Can you work these out from the model? Positions are in its coordinate system, mm. A direction names the side the tool comes from. Coordinates: 2 decimals unless noted, no trailing zeros. Order: outer loops, then holes, each group sorted by start corner. A loop starts at its lowest first (then second) coordinate and runs counter-clockwise, first axis right, second up. Notation, with made-up numbers: M -34,56.5 L 25,56.5 A33 ccw 25,92.5 Z; hole C 52,67 d3. An arc over 180 degrees is marked long. Answer as CSV lines item,"result". Start each with the question number.
1. If we mould it in two halves opening along Z, with no side actions, what happens to faces 1 (the face through (9.05, 16.44, -9.07)), 2 (the face through (0, 31, 0.794)), 3 (the face through (9.07, 16.44, 9.05)), 4 (the face through (2, 0, 0))? For each: released by +Z, released by -Z, zero draft, split by the parting line, or undercut.
2. On a 3-axis mill with a long thin cutter (end or side, diameter ignored), from which of +Z, -Z, +X, -X, +Y, -Y can I reach the whole of each face in a straight line? I mean faces 5 (the face through (2, 27, 4.762)), 6 (the face through (0, 31, -0.794)), 7 (the face through (-0.14, 1.22, -1.07)), 8 (the face through (-1.746, 11.668, 5.634)). Say none if no direction works.
3. Will these pins go through, and if not, where does the flat tip stop? pin 1 (10 mm diameter, centred on y = 15, z = -6.5, fed in from -X); pin 2 (3.5 mm diameter, centred on x = -1.5, y = 27.5, fed in from +Z); pin 3 (2 mm diameter, centred on y = 24.5, z = 1, fed in from -X).
4. If we section it at A-A (x = -7): List the corners of the cut face in (y, z) for me.
5. If we section it at C-C (z = 8.5): List the corners of the cut face in (x, y) for me.
6. I need wall thicknesses on line 1 along Y through (x, z) = (-4, 0); line 2 along Y through (x, z) = (0, 8.4); line 3 along Y through (x, z) = (7.75, 2.75). Which ranges of each line are inside material? Lowest first, please. Write a range as from..to.
```python
from build123d import *

# Parameters (mm, degrees)
SKETCH1_W               = 19.05
SKETCH1_H               = 19.05
EXTRUDE1_DEPTH          = 33.3375
CUT_EXTRUDE1_DEPTH      = 36.956086498
CUT_EXTRUDE1_DEPTH_BACK = 36.956086498
SKETCH2_R               = 1.7272
FILLET1_START           = 4.7625
FILLET1_OUTLINE_R       = 3.683
FILLET1_OUTLINE_R_2     = 1.7272
FILLET1_DEPTH           = 6.2375
FILLET1_START_2         = -0.79375
FILLET1_2_OUTLINE_R     = 3.683
FILLET1_2_OUTLINE_R_2   = 1.7272
FILLET1_2_DEPTH         = 1.5875
FILLET1_START_3         = 0.79375
FILLET1_3_OUTLINE_R     = 2.2352
FILLET1_3_OUTLINE_R_2   = 1.7272
FILLET1_3_DEPTH         = 3.96875
FILLET1_START_4         = -11
FILLET1_4_OUTLINE_R     = 1.0795
FILLET1_4_DEPTH         = 6.6947
FILLET1_START_5         = -9.525
FILLET1_5_DEPTH         = 19.05
FILLET1_START_6         = 16.48139325
FILLET1_6_OUTLINE_W     = 19.05
FILLET1_6_OUTLINE_H     = 1.5875
FILLET1_6_DEPTH         = 16.85610675
FILLET1_7_DEPTH         = 29.81639325
FILLET1_8_OUTLINE_R     = 1.0795
FILLET1_8_DEPTH         = 2.480030305
SPLIT1_DEPTH            = 33.3375


with BuildPart() as part:
    # Sketch1 → Extrude1 (new body)
    with BuildSketch(Plane(origin=(0, 0, 0), x_dir=(1, 0, 0), z_dir=(0, 1, 0))):
        Rectangle(SKETCH1_W, SKETCH1_H)
    extrude(amount=EXTRUDE1_DEPTH)

    # Sketch2 → Cut-Extrude1 (cut, two sides: drawn at the far end of the back side and taken through both)
    with BuildSketch(Plane.XY.offset(-CUT_EXTRUDE1_DEPTH_BACK)):
        with Locations((0, 28.3464)):
            Circle(SKETCH2_R)
    extrude(amount=CUT_EXTRUDE1_DEPTH + CUT_EXTRUDE1_DEPTH_BACK, mode=Mode.SUBTRACT)


with BuildPart() as body_2:
    # Sketch3 → Revolve1 (revolve)
    with BuildSketch(Plane.XY):
        with BuildLine():
            Line((12.168775296, 8.7376), (-12.7, 8.7376))
            Line((-12.7, 8.7376), (-12.7, 15.0876))
            Line((-12.7, 15.0876), (5.818775296, 15.0876))
            ThreePointArc((5.818775296, 15.0876), (10.308903356, 13.227728061), (12.168775296, 8.7376))
        make_face()
    revolve(axis=Axis((12.168775296, 8.7376, 0), (-1, 0, 0)))


with BuildPart() as part_1:
    add(part.part)

    # Combine1: cut body 2
    add(body_2.part, mode=Mode.SUBTRACT)

    # Fillet1: read off the stored shape, not the designer's step
    # Fillet1 outline → Fillet1 (cut)
    with BuildSketch(Plane.XY.offset(FILLET1_START)):
        with Locations((0, 28.3464)):
            Circle(FILLET1_OUTLINE_R)
        with Locations((0, 28.3464)):
            Circle(FILLET1_OUTLINE_R_2, mode=Mode.SUBTRACT)
    extrude(amount=FILLET1_DEPTH, mode=Mode.SUBTRACT)

    # Fillet1 2 outline → Fillet1 2 (cut)
    with BuildSketch(Plane.XY.offset(FILLET1_START_2)):
        with Locations((0, 28.3464)):
            Circle(FILLET1_2_OUTLINE_R)
        with Locations((0, 28.3464)):
            Circle(FILLET1_2_OUTLINE_R_2, mode=Mode.SUBTRACT)
    extrude(amount=FILLET1_2_DEPTH, mode=Mode.SUBTRACT)

    # Fillet1 3 outline → Fillet1 3 (cut)
    with BuildSketch(Plane.XY.offset(FILLET1_START_3)):
        with Locations((0, 28.3464)):
            Circle(FILLET1_3_OUTLINE_R)
        with Locations((0, 28.3464)):
            Circle(FILLET1_3_OUTLINE_R_2, mode=Mode.SUBTRACT)
    extrude(amount=FILLET1_3_DEPTH, mode=Mode.SUBTRACT)

    # Fillet1 4 outline → Fillet1 4 (cut)
    with BuildSketch(Plane.XY.offset(FILLET1_START_4)):
        with Locations((5.62102, 8.7376)):
            Circle(FILLET1_4_OUTLINE_R)
    extrude(amount=FILLET1_4_DEPTH, mode=Mode.SUBTRACT)

    # Fillet1 5 outline → Fillet1 5 (cut)
    with BuildSketch(Plane.YZ.offset(FILLET1_START_5)):
        with BuildLine():
            Line((33.3375, 0.79375), (24.881697256, 0.79375))
            ThreePointArc((24.881697256, 0.79375), (16.3449, 0), (24.881697256, -0.79375))
            Line((24.881697256, -0.79375), (33.3375, -0.79375))
            Line((33.3375, -0.79375), (33.3375, 0.79375))
        make_face()
    extrude(amount=FILLET1_5_DEPTH, mode=Mode.SUBTRACT)

    # Fillet1 6 outline → Fillet1 6 (cut)
    with BuildSketch(Plane(origin=(0, 0, 0), x_dir=(1, 0, 0), z_dir=(0, 1, 0)).offset(FILLET1_START_6)):
        Rectangle(FILLET1_6_OUTLINE_W, FILLET1_6_OUTLINE_H)
        with BuildLine():
            ThreePointArc((7.9375, 9.525), (9.060032015, 9.060032015), (9.525, 7.9375))
            Line((9.525, 7.9375), (9.525, 9.525))
            Line((9.525, 9.525), (7.9375, 9.525))
        make_face()
        with BuildLine():
            Line((9.525, -9.525), (9.525, -7.9375))
            ThreePointArc((9.525, -7.9375), (9.060032015, -9.060032015), (7.9375, -9.525))
            Line((7.9375, -9.525), (9.525, -9.525))
        make_face()
    extrude(amount=FILLET1_6_DEPTH, mode=Mode.SUBTRACT)

    # Fillet1 7 outline → Fillet1 7 (cut)
    with BuildSketch(Plane(origin=(0, 0, 0), x_dir=(1, 0, 0), z_dir=(0, 1, 0))):
        with BuildLine():
            ThreePointArc((7.9375, 9.525), (9.060032015, 9.060032015), (9.525, 7.9375))
            Line((9.525, 7.9375), (9.525, 9.525))
            Line((9.525, 9.525), (7.9375, 9.525))
        make_face()
        with BuildLine():
            Line((9.525, -9.525), (9.525, -7.9375))
            ThreePointArc((9.525, -7.9375), (9.060032015, -9.060032015), (7.9375, -9.525))
            Line((7.9375, -9.525), (9.525, -9.525))
        make_face()
    extrude(amount=FILLET1_7_DEPTH, mode=Mode.SUBTRACT)

    # Fillet1 8 outline → Fillet1 8 (cut)
    with BuildSketch(Plane(origin=(0, 0, 0), x_dir=(1, 0, 0), z_dir=(0, 1, 0))):
        Circle(FILLET1_8_OUTLINE_R)
    extrude(amount=FILLET1_8_DEPTH, mode=Mode.SUBTRACT)

    # Split1: read off the stored shape, not the designer's step
    # Split1 outline → Split1 (cut)
    with BuildSketch(Plane(origin=(0, 0, 0), x_dir=(1, 0, 0), z_dir=(0, 1, 0))):
        with BuildLine():
            Line((-9.525, 9.525), (-9.525, 0))
            ThreePointArc((-9.525, 0), (-6.735192091, 6.735192091), (0, 9.525))
            Line((0, 9.525), (-9.525, 9.525))
        make_face()
        with BuildLine():
            ThreePointArc((0, -9.525), (-6.735192091, -6.735192091), (-9.525, 0))
            Line((-9.525, 0), (-9.525, -9.525))
            Line((-9.525, -9.525), (0, -9.525))
        make_face()
    extrude(amount=SPLIT1_DEPTH, mode=Mode.SUBTRACT)


solid = part_1.part
```
Solved:
1,face 1,"released by -Z"
1,face 2,"undercut"
1,face 3,"released by +Z"
1,face 4,"zero draft"
2,face 5,"+Z"
2,face 6,"+X, -X, +Y"
2,face 7,"-Y"
2,face 8,"-X"
3,pin 1,"x = -9.41"
3,pin 2,"z = 4.76"
3,pin 3,"x = -9.49"
4,outline,"M 0,-6.46 L 33.34,-6.46 L 33.34,-0.79 L 24.88,-0.79 A4.31 cw long 24.88,0.79 L 33.34,0.79 L 33.34,6.46 L 0,6.46 Z; hole C 8.74,0 d12.7"
5,outline,"M -4.3,0 L 9.42,0 L 9.42,33.34 L -4.3,33.34 Z; hole C 0,28.35 d7.37"
6,line 1,"0..2.39, 15.09..16.34"
6,line 2,"0..24.66, 32.03..33.34"
6,line 3,"0..3.35, 14.13..17.34, 23.96..33.34"
